from build123d import *

# Parameters (mm, degrees)
F0_R     = 2.5
F1_DEPTH = 12


with BuildPart() as f1:
    # F0 (on Front) → F1 (new body)
    with BuildSketch(Plane.XZ):
        with BuildLine():
            Line((0, 80), (0, 0))
            Line((0, 0), (100, 0))
            Line((100, 0), (100, 50))
            Line((100, 50), (50, 80))
            Line((50, 80), (26, 80))
            Line((26, 80), (41.692823, 56.83966))
            ThreePointArc((41.692823, 56.83966), (41.824435, 53.290779), (38.274518, 53.190937))
            Line((38.274518, 53.190937), (37.685428, 54.055142))
            Line((37.685428, 54.055142), (20, 80))
            Line((20, 80), (0, 80))
        make_face()
        with Locations((10, 10)):
            Circle(F0_R, mode=Mode.SUBTRACT)
        with Locations((60, 10)):
            Circle(F0_R, mode=Mode.SUBTRACT)
    extrude(amount=F1_DEPTH)


solid = f1.part
Here's how the part is built. I have some questions about the finished solid (model axes, mm). A direction names the side the tool comes from. Give positions to 0.01 mm unless a question says otherwise; leave off trailing zeros. Loops run counter-clockwise (first coordinate to the right, second up) from the corner with the lowest first, then second, coordinate; pieces in that order, holes last. Notation, with made-up numbers: (53, -18) -> (104, -18) arc R28 cw to (104, 10) -> close; hole circle Ø1 at (29.5, 0). An arc over 180 degrees is marked (long way). Answer as a JSON object with one key per item and string values. Group by question number.
Item 1: Imagine slicing it at C-C on y = -9. Write out the boundary of the cut face in (x, z), then the cut area to 3 significant figures.
Item 2: Will these pins go through, and if not, where does the flat tip stop? pin 1 (12 mm diameter, centred on x = 59, z = 19.5, fed in from +Y); pin 2 (4.5 mm diameter, centred on x = 10, z = 10, fed in from -Y); pin 3 (4 mm diameter, centred on y = -8.5, z = 55, fed in from +X); pin 4 (6 mm diameter, centred on x = 79, y = -5, fed in from +Z).
Item 3: Imagine slicing it at D-D on z = 69. Write out the boundary of the cut face in (x, y).
Item 4: Thinking about a two-plate mould opening in X: for faces 1 (the cylindrical face through (41.86, -5.92, 53.33)), 2 (the flat face through (10, -6, 80)), 3 (the flat face through (0, -6, 41)), which applies, pulls with the +X half, pulls with the -X half, needs draft (parallel to the pull), parting line crosses it, or undercut?
Item 5: Imagine slicing it at B-B on x = 10. Write out the boundary of the cut face in (y, z).
Item 6: I need wall thicknesses on L1, parallel to Z at x = 10, y = -3.25; L2, parallel to X at y = -4.25, z = 9; L3, parallel to Z at x = 60, y = -3.5. Which ranges of each line are inside material? Lowest first, please.
Item 7: Imagine slicing it at A-A on z = 10. Write out the boundary of the cut face in (x, y), then the cut area to 3 significant figures.
Item 8: On a 3-axis mill with a long thin cutter (end or side, diameter ignored), from which of +Z, -Z, +X, -X, +Y, -Y can I reach the whole of each face in a straight line? I mean faces 4 (the flat face through (33.74, -5.92, 68.58)), 5 (the flat face through (38, -6, 80)). Say none if no direction works.
Answer list:
{
 "1": {"outline": "(0, 0) -> (100, 0) -> (100, 50) -> (50, 80) -> (26, 80) -> (41.69, 56.84) arc R2.5 cw (long way) to (38.27, 53.19) -> (37.69, 54.06) -> (20, 80) -> (0, 80) -> close; hole circle Ø5 at (10, 10); hole circle Ø5 at (60, 10)", "area": "7,050 mm2"},
 "2": {"pin 1": "stops at y = 0", "pin 2": "passes through", "pin 3": "stops at x = 95", "pin 4": "stops at z = 64.4"},
 "3": {"outline": "(0, -12) -> (27.5, -12) -> (27.5, 0) -> (0, 0) -> close; (33.45, -12) -> (68.33, -12) -> (68.33, 0) -> (33.45, 0) -> close"},
 "4": {"face 1": "undercut", "face 2": "needs draft", "face 3": "pulls with the -X half"},
 "5": {"outline": "(-12, 0) -> (0, 0) -> (0, 7.5) -> (-12, 7.5) -> close; (-12, 12.5) -> (0, 12.5) -> (0, 80) -> (-12, 80) -> close"},
 "6": {"L1": "z = 0 to 7.5, 12.5 to 80", "L2": "x = 0 to 7.71, 12.29 to 57.71, 62.29 to 100", "L3": "z = 0 to 7.5, 12.5 to 74"},
 "7": {"outline": "(0, -12) -> (7.5, -12) -> (7.5, 0) -> (0, 0) -> close; (12.5, -12) -> (57.5, -12) -> (57.5, 0) -> (12.5, 0) -> close; (62.5, -12) -> (100, -12) -> (100, 0) -> (62.5, 0) -> close", "area": "1,080 mm2"},
 "8": {"face 4": "+Y, -Y", "face 5": "+Z, +X, -X, +Y, -Y"}
}
